Source: three-view drawing plus pictorial views. Frame: mm from the lowest corner of the part. Give positions to 0.01 mm unless a question says otherwise; leave off trailing zeros. Loops run counter-clockwise (first coordinate to the right, second up) from the corner with the lowest first, then second, coordinate; pieces in that order, holes last. Notation, with made-up numbers: (39.25, -15) - (56.25, -15) arc R26 ccw to (56.25, 7) - close; hole circle Ø4 at (4.25, 42.25). An arc over 180 degrees is marked (long way). Put each result on its own line as item: value.
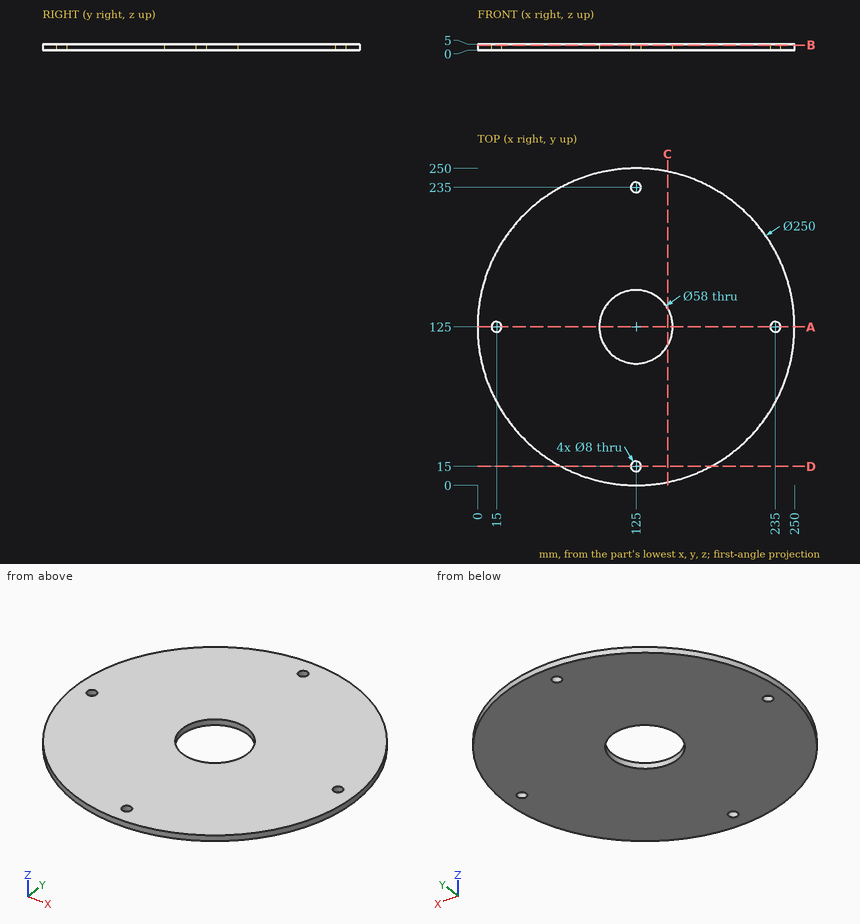
1) Section query C-C, the plane x = 150. Output: boundary loops of the cut face in (y, z).
Check result:
outline: (2.53, 0) - (110.3, 0) - (110.3, 5) - (2.53, 5) - close; (139.7, 0) - (247.47, 0) - (247.47, 5) - (139.7, 5) - close
2) Pin query (flat end, axial travel): P1, Ø1.5, axis at y = 141.5, z = 2, coming from the +X side; P2, Ø6.5, axis at x = 15, y = 125, coming from the -Z side; P3, Ø1, axis at y = 88, z = 4, coming from the -X side; P4, Ø3, axis at y = 217, z = 2.5, coming from the +X side (3 decimals). Return the tip coordinate at first contact, or that it passes through.
Check result:
P1: x = 249
P2: through
P3: x = 5.45
P4: x = 211.225
3) Section query D-D, the plane y = 15. Output: boundary loops of the cut face in (x, z), plus the area to 3 significant figures.
Check result:
outline: (65.63, 0) - (121, 0) - (121, 5) - (65.63, 5) - close; (129, 0) - (184.37, 0) - (184.37, 5) - (129, 5) - close
area: 554 mm²
4) Section query B-B, the plane z = 4.2. Output: boundary loops of the cut face in (x, y), plus the area to 3 significant figures.
Check result:
outline: circle Ø250 at (125, 125); hole circle Ø8 at (15, 125); hole circle Ø58 at (125, 125); hole circle Ø8 at (125, 15); hole circle Ø8 at (125, 235); hole circle Ø8 at (235, 125)
area: 46,200 mm²
5) Material intervals for line 1 along Y through (x, z) = (125, 1.95); line 2 along Y through (x, z) = (150, 4.45); line 3 along Y through (x, z) = (15, 2.6), sorted ascending. Write a range as [from, to].
Check result:
line 1: [0, 11], [19, 96], [154, 231], [239, 250]
line 2: [2.53, 110.3], [139.7, 247.47]
line 3: [65.63, 121], [129, 184.37]
6) Section query A-A, the plane y = 125. Output: boundary loops of the cut face in (x, z).
Check result:
outline: (0, 0) - (11, 0) - (11, 5) - (0, 5) - close; (19, 0) - (96, 0) - (96, 5) - (19, 5) - close; (154, 0) - (231, 0) - (231, 5) - (154, 5) - close; (239, 0) - (250, 0) - (250, 5) - (239, 5) - close
